from build123d import *

# Parameters (mm, degrees)
SKETCH_1_W          = 40
SKETCH_1_H          = 30
EXTRUDE_1_DEPTH     = 50
SKETCH_2_R          = 2.55
CUT_EXTRUDE_1_DEPTH = 64.496259876
SKETCH_3_R          = 4.5
CUT_EXTRUDE_2_DEPTH = 20
SKETCH_4_R          = 2.55
CUT_EXTRUDE_3_DEPTH = 59.417154289
SKETCH_5_W          = 9
SKETCH_5_H          = 4.5
CUT_EXTRUDE_4_DEPTH = 15
SKETCH_7_W          = 40
SKETCH_7_H          = 30.941216598
CUT_EXTRUDE_5_DEPTH = 20
FILLET_1_R          = 10
FILLET_2_R          = 2


with BuildPart() as part:
    # 草图1 → 凸台-拉伸1 (new body)
    with BuildSketch(Plane(origin=(0, 0, 0), x_dir=(1, 0, 0), z_dir=(0, 1, 0))):
        with Locations((5.135135135, 1.756756757)):
            Rectangle(SKETCH_1_W, SKETCH_1_H)
    extrude(amount=EXTRUDE_1_DEPTH)

    # 草图2 → 切除-拉伸1 (cut, through all)
    with BuildSketch(Plane.XY.offset(13.243243243)):
        with Locations((-4.864864865, 10)):
            Circle(SKETCH_2_R)
        with Locations((15.135135135, 10)):
            Circle(SKETCH_2_R)
    extrude(amount=-CUT_EXTRUDE_1_DEPTH, mode=Mode.SUBTRACT)

    # 草图3 → 切除-拉伸2 (cut)
    with BuildSketch(Plane.XY.offset(13.243243243)):
        with Locations((-4.864864865, 10)):
            Circle(SKETCH_3_R)
        with Locations((15.135135135, 10)):
            Circle(SKETCH_3_R)
    extrude(amount=-CUT_EXTRUDE_2_DEPTH, mode=Mode.SUBTRACT)

    # 草图4 → 切除-拉伸3 (cut, through all)
    with BuildSketch(Plane(origin=(0, 50, 0), x_dir=(1, 0, 0), z_dir=(0, 1, 0))):
        with Locations(Location((5.135135135, -3.243243243, 0), (0, 0, 270))):
            Circle(SKETCH_4_R)
    extrude(amount=-CUT_EXTRUDE_3_DEPTH, mode=Mode.SUBTRACT)

    # 草图5 → 切除-拉伸4 (cut)
    with BuildSketch(Plane.XY.offset(13.243243243)):
        with Locations((5.135135135, 39.75)):
            Rectangle(SKETCH_5_W, SKETCH_5_H)
    extrude(amount=-CUT_EXTRUDE_4_DEPTH, mode=Mode.SUBTRACT)

    # 草图7 → 切除-拉伸5 (cut)
    with BuildSketch(Plane.XY.offset(13.243243243)):
        with Locations((5.135135135, 15.470608299)):
            Rectangle(SKETCH_7_W, SKETCH_7_H)
    extrude(amount=-CUT_EXTRUDE_5_DEPTH, mode=Mode.SUBTRACT)

    # 圆角1
    # the kernel refuses this fillet: 10 mm, written as the material it adds along each edge
    with BuildSketch(Plane(origin=(25.135135135, 30.941216598, -6.756756757), x_dir=(0, 0, 1), z_dir=(-1, 0, 0))) as fillet_1_piece_1_section:
        with BuildLine():
            CenterArc((FILLET_1_R, -FILLET_1_R), FILLET_1_R, 90, 90)
            Line((0, -FILLET_1_R), (0, 0))
            Line((0, 0), (FILLET_1_R, 0))
        make_face()
    fillet_1_piece_1 = extrude(amount=40, mode=Mode.PRIVATE)
    fillet_1_piece_1 = fillet_1_piece_1 - Plane(origin=(5.135135135, 28.670722108, 3.243243243), x_dir=(0, 0, 1), z_dir=(0, 1, 0)) * Cylinder(2.55, 120, mode=Mode.PRIVATE)
    add(fillet_1_piece_1)

    # 圆角2
    fillet_2_edges = [part.edges().sort_by_distance(p)[0] for p in [
        (25.135135135, 50, -1.756756757),
        (-14.864864865, 50, -1.756756757),
        (-14.864864865, 0, -11.756756757),
        (25.135135135, 0, -11.756756757),
    ]]
    fillet(fillet_2_edges, radius=FILLET_2_R)


solid = part.part
Input: part model. Units: mm. Frame: model coordinates. A direction names the side the tool comes from. Coordinates: 2 decimals unless noted, no trailing zeros. Loops run counter-clockwise (first coordinate to the right, second up) from the corner with the lowest first, then second, coordinate; pieces in that order, holes last.
(1) Section A-A on y = 10. Return the cut outline in (x, z).
(2) Section D-D on z = 5. Return the cut outline in (x, y).
(3) Material intervals for probe 1 along Y at (x, z) = (7, 6.5); probe 2 along Z at (x, y) = (19, 14.5); probe 3 along X at (y, z) = (40, 3.5), sorted ascending.
(4) First-contact query: pin 1 Ø1.5 at (x, y) = (12.5, 17.5) entering from +Z; pin 2 Ø1 at (x, z) = (9.5, 2) entering from -Y; pin 3 Ø8 at (x, z) = (8, 6.5) entering from -Y; pin 4 Ø4 at (x, y) = (-4.86, 10) entering from -Z. Flat tips, straight axial feed; report the tip coordinate or a pass-through.
(5) Section C-C on x = 16. Return the cut outline in (y, z), then the cut area to 3 significant figures.
(6) Pull-direction query (Z, two-part tool) for faces 4 (the face through (5.901, 46.056, 5.675)), 5 (the face through (5, 40, -1.757)), 6 (the face through (9.635, 40, 6)); classes: released by +Z, released by -Z, zero draft, split by the parting line, or undercut.
(7) Set-up query: faces 1 (the face through (5, 37.5, 6)), 2 (the face through (5, 25, -16.757)), 3 (the face through (5, 30.941, 8)). Return all of +Z, -Z, +X, -X, +Y, -Y with unobstructed straight access to the full face (end or side cutting, diameter ignored); none if empty.
(8) Section B-B on z = -13. Return the cut outline in (x, y), then the cut area to 3 significant figures.
Data:
1. outline: (-14.86, -16.76) - (-7.41, -16.76) - (-7.41, -6.76) - (-14.86, -6.76) - close; (-2.31, -16.76) - (12.59, -16.76) - (12.59, -6.76) - (-2.31, -6.76) - close; (17.69, -16.76) - (25.14, -16.76) - (25.14, -6.76) - (17.69, -6.76) - close
2. outline: (-14.86, 30.94) - (3.29, 30.94) - (3.29, 37.5) - (0.64, 37.5) - (0.64, 42) - (3.29, 42) - (3.29, 50) - (-12.86, 50) arc R2 ccw to (-14.86, 48) - close; (6.98, 30.94) - (25.14, 30.94) - (25.14, 48) arc R2 ccw to (23.14, 50) - (6.98, 50) - (6.98, 42) - (9.64, 42) - (9.64, 37.5) - (6.98, 37.5) - close
3. probe 1: y = 30.94 to 37.5, 42 to 50
3. probe 2: z = -16.76 to -6.76
3. probe 3: x = -14.86 to 0.64, 9.64 to 25.14
4. pin 1: stops at z = -6.76
4. pin 2: stops at y = 30.79
4. pin 3: stops at y = 30.91
4. pin 4: passes through
5. outline: (0, -16.76) - (7.6, -16.76) - (7.6, -6.76) - (0, -6.76) - close; (12.4, -16.76) - (50, -16.76) - (50, 13.24) - (30.94, 13.24) - (30.94, 3.24) arc R10 cw to (20.94, -6.76) - (12.4, -6.76) - close
5. area: 855 mm2
6. face 4: undercut
6. face 5: released by +Z
6. face 6: zero draft
7. face 1: +Z
7. face 2: -Z, +X, -X, +Y, -Y
7. face 3: +Z, +X, -X, -Y
8. outline: (-14.86, 2) arc R2 ccw to (-12.86, 0) - (23.14, 0) arc R2 ccw to (25.14, 2) - (25.14, 48) arc R2 ccw to (23.14, 50) - (-12.86, 50) arc R2 ccw to (-14.86, 48) - close; hole circle Ø5.1 at (-4.86, 10); hole circle Ø5.1 at (15.14, 10)
8. area: 1,960 mm2
